```python
from build123d import *

# Parameters (mm, degrees)
F1_DEPTH = 25
F2_DEPTH = 25


# Not quite as in the source:
# - ends of sketch curves that miss each other by under 0.0002 mm in the source are joined
# - the dataset's text gives a spline's control points without its knots; the knots are read off the source's solid


with BuildPart() as f1:
    # F0 (on Front) → F1 (new body)
    with BuildSketch(Plane.XZ):
        with BuildLine():
            Line((-22.0594022245, 9.6566297112), (-67.6395371556, 9.6566297112))
            Line((-67.6395371556, 9.6566297112), (-67.6395371556, -10.3433702888))
            Line((-67.6395371556, -10.3433702888), (-7.6395371556, -10.3433702888))
            Line((-7.6395371556, -10.3433702888), (-7.6395371556, 9.6566297112))
            Line((-7.6395371556, 9.6566297112), (-15.8638085328, 9.6566297112))
            add(Edge.make_bspline(
                [(-15.872090736, 9.6453477446), (-15.8693299564, 9.6491085329), (-15.866569222, 9.6528691885), (-15.8638085328, 9.6566297112)],
                knots=[0.0211094133, 0.0211094133, 0.0211094133, 0.0211094133, 0.0211910509, 0.0211910509, 0.0211910509, 0.0211910509], degree=3))
            Line((-15.872090736, 9.6453477446), (-22.0594022245, 9.6566297112))
        make_face()
    extrude(amount=F1_DEPTH)

    # F2 (add): a face of the model
    f2_faces = [f1.faces().sort_by_distance(p)[0] for p in [
        (-18.9657464803, -12.5, 9.6509887279),
    ]]
    extrude(f2_faces, amount=F2_DEPTH)


solid = f1.part
```
Geometry: final body of the model. Coordinates: model frame, mm. A direction names the side the tool comes from. Round coordinates to 2 decimals unless told otherwise and drop trailing zeros. Loops run counter-clockwise (first coordinate to the right, second up) from the corner with the lowest first, then second, coordinate; pieces in that order, holes last.
Item 1: Section B-B, the plane z = 28. Output: boundary loops of the cut face in (x, y), plus the area to 3 significant figures.
Checked values:
outline: (-22.03, -25) - (-15.84, -25) - (-15.84, 0) - (-22.03, 0) - close
area: 155 mm2
Item 2: Reachability of faces 1 (the flat face through (-45, -12, 9.657)), 2 (the flat face through (-12, -12, 9.657)), 3 (the flat face through (-38, -12, -10.343)) from +Z, -Z, +X, -X, +Y, -Y: full face, straight path, thin tool, end or side. Return the list, or none.
Checked values:
face 1: +Z, -X, +Y, -Y
face 2: +Z, +X, +Y, -Y
face 3: -Z, +X, -X, +Y, -Y
Item 3: Contact query for flat-ended pins moving along their axis: P1, Ø5, axis at y = -22.5, z = 23.5, coming from the -X side; P2, Ø2.5, axis at x = -13.5, y = -18, coming from the +Z side; P3, Ø5, axis at y = -13.5, z = 13, coming from the -X side. Output: stop coordinate, or through.
Checked values:
P1: stops at x = -22.04
P2: stops at z = 9.66
P3: stops at x = -22.06
Item 4: Section A-A, the plane x = -36. Output: boundary loops of the cut face in (y, z).
Checked values:
outline: (-25, -10.34) - (0, -10.34) - (0, 9.66) - (-25, 9.66) - close
Item 5: Line query: L1, parallel to X at y = -12, z = 16; L2, parallel to Z at x = -65, y = -3; L3, parallel to Z at x = -16.5, y = -13. Output: solid intervals per line, ascending.
Checked values:
L1: x = -22.05 to -15.86
L2: z = -10.34 to 9.66
L3: z = -10.34 to 34.65
